Read the model definition and answer for the solid it produces. Units are mm, in the model's axes. A direction names the side the tool comes from. Give positions to 0.01 mm unless a question says otherwise; leave off trailing zeros. Write each loop counter-clockwise with the first axis right and the second up, starting at its lowest first coordinate (ties: lowest second). Pieces come first, ordered by that corner, then holes. Notation, with made-up numbers: M -29,47 L 30,47 A26 ccw 30,76 Z; hole C 15.25,-36.5 d1. An arc over 180 degrees is marked long. Use a Markdown table: item, result. Add a question column.
Item 1: Consider probe 1 along X at (y, z) = (-19, 4.75); probe 2 along Y at (x, z) = (0, 2.5) (3 decimals); probe 3 along Y at (x, z) = (-0.5, 1.75) (3 decimals). Determine where each line is inside the solid, lowest interval first. Write a range as [from, to].
Item 2: A cutting plane is placed at D-D on x = 21. Determine the outline of the cut face in (y, z) (3 decimals), then the cut area to 3 significant figures.
Item 3: A cutting plane is placed at B-B on y = -14.5. Determine the outline of the cut face in (x, z), then the cut area to 3 significant figures.
Item 4: A cutting plane is placed at A-A on x = 0. Determine the outline of the cut face in (y, z) (3 decimals).
Item 5: The mould has two halves that part along Y. Classify faces 4 (the flat face through (-17, -15, 3)), 5 (the cylindrical face through (-18.167, 27.095, 4.93)), 6 (the cylindrical face through (0.055, -21.334, 1.479)), 7 (the flat face through (0, -6, 0)): pulls with the +Y half, pulls with the -Y half, needs draft (parallel to the pull), parting line crosses it, or undercut.
Item 6: Given P1, Ø10, axis at x = 2.5, y = -13, coming from the +Z side; P2, Ø3, axis at x = -18, y = -15, coming from the +Z side; P3, Ø1.5, axis at x = 19.5, z = 6.5, coming from the +Y side, each flat-ended and moving along its own axis, determine where each tip first touches the part or whether it passes through.
Item 7: A cutting plane is placed at C-C on z = 5.75. Determine the outline of the cut face in (x, y) (3 decimals).
Item 8: For faces 1 (the flat face through (24.236, 21.579, 4.93)), 2 (the flat face through (4.6, -15, 6)), 3 (the cylindrical face through (-20.055, -9.536, 1.479)), determine the directions among +Z, -Z, +X, -X, +Y, -Y from which every point of the face is accessible in a straight line to the end or side of a thin tool.
from build123d import *

# Parameters (mm, degrees)
F0_R     = 8.05
F1_DEPTH = 10
F2_DEPTH = 3


# Not quite as in the source:
# - ends of sketch curves that miss each other by under 0.0002 mm in the source are joined


with BuildPart() as f1:
    # F0 (on Top) → F1 (new body)
    with BuildSketch(Plane.XY):
        with BuildLine():
            ThreePointArc((-16.278933, 27.465), (-18.1923501618, 27.0843976626), (-19.8144669059, 26.0005339059))
            Line((-19.8144669059, 26.0005339059), (-28.535534, 17.279466))
            ThreePointArc((-28.535534, 17.279466), (-29.6193976626, 15.6573491618), (-30, 13.743932))
            Line((-30, 13.743932), (-30, -25.965))
            ThreePointArc((-30, -25.965), (-29.5606601718, -27.0256601718), (-28.5, -27.465))
            Line((-28.5, -27.465), (28.5, -27.465))
            ThreePointArc((28.5, -27.465), (29.5606601718, -27.0256601718), (30, -25.965))
            Line((30, -25.965), (30, 13.743932))
            ThreePointArc((30, 13.743932), (29.6193976626, 15.6573491618), (28.5355339059, 17.2794659059))
            Line((28.5355339059, 17.2794659059), (19.814466, 26.000533))
            ThreePointArc((19.814466, 26.000533), (18.1923494885, 27.0843975273), (16.278932, 27.465))
            Line((16.278932, 27.465), (-16.278933, 27.465))
        make_face()
        with BuildLine():
            ThreePointArc((-24.6, -12.035), (-20, -7.435), (-15.4, -12.035))
            Line((-15.4, -12.035), (-15.4, -18.835))
            ThreePointArc((-15.4, -18.835), (-20, -23.435), (-24.6, -18.835))
            Line((-24.6, -18.835), (-24.6, -12.035))
        make_face(mode=Mode.SUBTRACT)
        with BuildLine():
            ThreePointArc((4.6, -18.835), (0, -23.435), (-4.6, -18.835))
            Line((-4.6, -18.835), (-4.6, -12.035))
            ThreePointArc((-4.6, -12.035), (0, -7.435), (4.6, -12.035))
            Line((4.6, -12.035), (4.6, -18.835))
        make_face(mode=Mode.SUBTRACT)
        with BuildLine():
            ThreePointArc((15.4, -12.035), (20, -7.435), (24.6, -12.035))
            Line((24.6, -12.035), (24.6, -18.835))
            ThreePointArc((24.6, -18.835), (20, -23.435), (15.4, -18.835))
            Line((15.4, -18.835), (15.4, -12.035))
        make_face(mode=Mode.SUBTRACT)
        with Locations((0, 4.965)):
            Circle(F0_R, mode=Mode.SUBTRACT)
    extrude(amount=F1_DEPTH)

    # F0 (on Top) → F2 (join)
    with BuildSketch(Plane.XY):
        with BuildLine():
            Line((-15.4, -18.835), (-15.4, -12.035))
            ThreePointArc((-15.4, -12.035), (-20, -7.435), (-24.6, -12.035))
            Line((-24.6, -12.035), (-24.6, -18.835))
            ThreePointArc((-24.6, -18.835), (-20, -23.435), (-15.4, -18.835))
        make_face()
        with BuildLine():
            ThreePointArc((-17.5, -18.835), (-20, -21.335), (-22.5, -18.835))
            Line((-22.5, -18.835), (-22.5, -12.035))
            ThreePointArc((-22.5, -12.035), (-20, -9.535), (-17.5, -12.035))
            Line((-17.5, -12.035), (-17.5, -18.835))
        make_face(mode=Mode.SUBTRACT)
        with BuildLine():
            Line((-4.6, -12.035), (-4.6, -18.835))
            ThreePointArc((-4.6, -18.835), (0, -23.435), (4.6, -18.835))
            Line((4.6, -18.835), (4.6, -12.035))
            ThreePointArc((4.6, -12.035), (0, -7.435), (-4.6, -12.035))
        make_face()
        with BuildLine():
            ThreePointArc((2.5, -18.835), (0, -21.335), (-2.5, -18.835))
            Line((-2.5, -18.835), (-2.5, -12.035))
            ThreePointArc((-2.5, -12.035), (0, -9.535), (2.5, -12.035))
            Line((2.5, -12.035), (2.5, -18.835))
        make_face(mode=Mode.SUBTRACT)
        with BuildLine():
            Line((24.6, -18.835), (24.6, -12.035))
            ThreePointArc((24.6, -12.035), (20, -7.435), (15.4, -12.035))
            Line((15.4, -12.035), (15.4, -18.835))
            ThreePointArc((15.4, -18.835), (20, -23.435), (24.6, -18.835))
        make_face()
        with BuildLine():
            ThreePointArc((22.5, -18.835), (20, -21.335), (17.5, -18.835))
            Line((17.5, -18.835), (17.5, -12.035))
            ThreePointArc((17.5, -12.035), (20, -9.535), (22.5, -12.035))
            Line((22.5, -12.035), (22.5, -18.835))
        make_face(mode=Mode.SUBTRACT)
    extrude(amount=F2_DEPTH)


solid = f1.part
Filled in:
| question | item | result |
|---|---|---|
| 1 | probe 1 | [-30, -24.6], [-15.4, -4.6], [4.6, 15.4], [24.6, 30] |
| 1 | probe 2 | [-27.465, -21.335], [-9.535, -3.085], [13.015, 27.465] |
| 1 | probe 3 | [-27.465, -21.284], [-9.586, -3.069], [12.999, 27.465] |
| 2 | outline | M -27.465,0 L -21.126,0 L -21.126,3 L -23.325,3 L -23.325,10 L -27.465,10 Z; M -9.744,0 L 24.815,0 L 24.815,10 L -7.545,10 L -7.545,3 L -9.744,3 Z |
| 2 | area | 378 mm² |
| 3 | outline | M -30,0 L -22.5,0 L -22.5,3 L -24.6,3 L -24.6,10 L -30,10 Z; M -17.5,0 L -2.5,0 L -2.5,3 L -4.6,3 L -4.6,10 L -15.4,10 L -15.4,3 L -17.5,3 Z; M 2.5,0 L 17.5,0 L 17.5,3 L 15.4,3 L 15.4,10 L 4.6,10 L 4.6,3 L 2.5,3 Z; M 22.5,0 L 30,0 L 30,10 L 24.6,10 L 24.6,3 L 22.5,3 Z |
| 3 | area | 362 mm² |
| 4 | outline | M -27.465,0 L -21.335,0 L -21.335,3 L -23.435,3 L -23.435,10 L -27.465,10 Z; M -9.535,0 L -3.085,0 L -3.085,10 L -7.435,10 L -7.435,3 L -9.535,3 Z; M 13.015,0 L 27.465,0 L 27.465,10 L 13.015,10 Z |
| 5 | face 4 | undercut |
| 5 | face 5 | pulls with the +Y half |
| 5 | face 6 | undercut |
| 5 | face 7 | needs draft |
| 6 | P1 | z = 10 |
| 6 | P2 | z = 3 |
| 6 | P3 | y = 26.81 |
| 7 | outline | M -30,-25.965 A1.5 ccw -28.5,-27.465 L 28.5,-27.465 A1.5 ccw 30,-25.965 L 30,13.744 A5 ccw 28.536,17.279 L 19.814,26.001 A5 ccw 16.279,27.465 L -16.279,27.465 A5 ccw -19.814,26.001 L -28.536,17.279 A5 ccw -30,13.744 Z; hole M -24.6,-18.835 A4.6 ccw -15.4,-18.835 L -15.4,-12.035 A4.6 ccw -24.6,-12.035 Z; hole C 0,4.965 d16.1; hole M -4.6,-18.835 A4.6 ccw 4.6,-18.835 L 4.6,-12.035 A4.6 ccw -4.6,-12.035 Z; hole M 15.4,-18.835 A4.6 ccw 24.6,-18.835 L 24.6,-12.035 A4.6 ccw 15.4,-12.035 Z |
| 8 | face 1 | +Z, -Z, +X, +Y |
| 8 | face 2 | +Z |
| 8 | face 3 | +Z, -Z |
